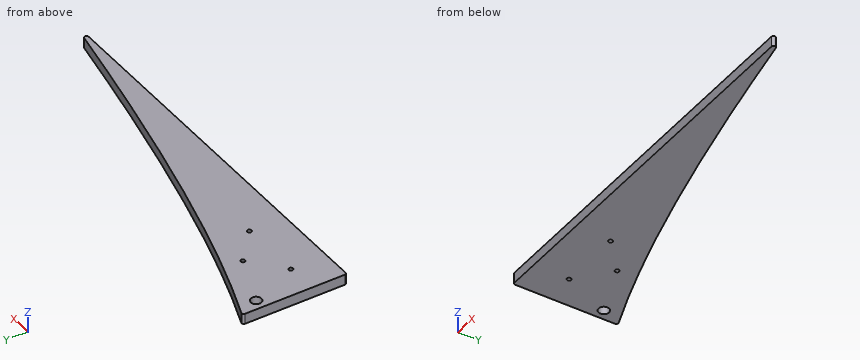
```python
from build123d import *

# Parameters (mm, degrees)
SKETCH1_R           = 6.35
BOSS_EXTRUDE1_DEPTH = 12.7
FILLET1_R           = 2.54
FILLET2_R           = 2.54
SKETCH2_R           = 2.54
CUT_EXTRUDE1_DEPTH  = 203.2


with BuildPart() as part:
    # Sketch1 → Boss-Extrude1 (new body)
    with BuildSketch(Plane.XY):
        with BuildLine():
            Line((0, 0), (0, 127))
            add(Edge.make_bspline(
                [(0, 127), (169.846972044, 59.080713691), (508, 0)],
                knots=[0, 0, 0, 1, 1, 1], degree=2))
            Line((508, 0), (0, 0))
        make_face()
        with Locations((12.7, 101.6)):
            Circle(SKETCH1_R, mode=Mode.SUBTRACT)
    extrude(amount=BOSS_EXTRUDE1_DEPTH)

    # Fillet1
    fillet1_edges = [part.edges().sort_by_distance(p)[0] for p in [
        (0, 127, 6.35),
    ]]
    fillet(fillet1_edges, radius=FILLET1_R)

    # Fillet2
    fillet2_edges = [part.edges().sort_by_distance(p)[0] for p in [
        (0, 0, 6.35),
        (508, 0, 6.35),
    ]]
    fillet(fillet2_edges, radius=FILLET2_R)

    # Sketch2 → Cut-Extrude1 (cut)
    with BuildSketch(Plane.XY.offset(12.7)):
        with Locations((76.2, 76.2)):
            Circle(SKETCH2_R)
        with Locations((37.70884, 43.20032)):
            Circle(SKETCH2_R)
        with Locations((114.69116, 43.20032)):
            Circle(SKETCH2_R)
    extrude(amount=-CUT_EXTRUDE1_DEPTH, mode=Mode.SUBTRACT)


solid = part.part
```
The listing builds one solid part. Answer for the finished solid, in the listing's coordinates (mm). Give positions to 0.01 mm unless a question says otherwise; leave off trailing zeros. Answer as a JSON object with one key per item and string values. Group by question number.
Item 1: Flat-ended cylindrical pins translate along their axes: pin 1 (8 mm diameter, centred on x = 114.69, y = 43.2, fed in from -Z); pin 2 (5 mm diameter, centred on x = 347, z = 1.5, fed in from +Y); pin 3 (4 mm diameter, centred on x = 426, z = 3.5, fed in from +Y). Find the tip coordinate at first contact, or state that the pin passes through.
Item 2: Consider L1, parallel to Y at x = 12.7, z = 9.5; L2, parallel to Y at x = 76.2, z = 5.25; L3, parallel to Y at x = 285.5, z = 8.75. Determine where each line is inside the solid, lowest interval first. Write a range as from..to.
Item 3: The part is cut by section A-A on z = 7.5. Give the number of separate pieces and of enclosed holes in the cut face, and give its area (3 significant figures).
Result set:
{
 "1": {"pin 1": "z = 0", "pin 2": "y = 31.12", "pin 3": "y = 15.31"},
 "2": {"L1": "0..95.25, 107.95..122.02", "L2": "0..73.66, 78.74..99.69", "L3": "0..43.87"},
 "3": {"separate pieces": "1", "enclosed holes": "4", "area": "27,700 mm²"}
}
